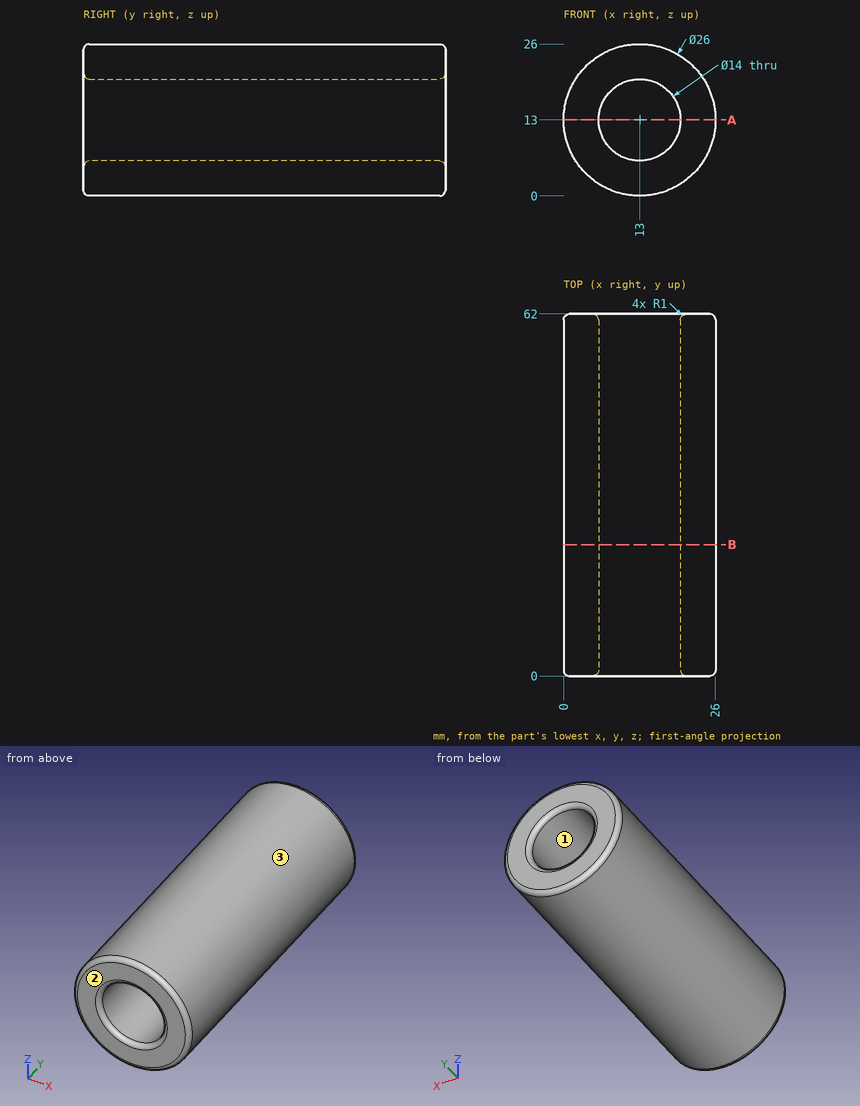
The figure shows three views and two pictorial views of one solid part (mm, origin at its lowest corner). Answer the questions. Coordinates: 2 decimals unless noted, no trailing zeros. Order: outer loops, then holes, each group sorted by start corner. A loop starts at its lowest first (then second) coordinate and runs counter-clockwise, first axis right, second up. Notation, with made-up numbers: M 89.25,-36 L 109.25,-36 A29 cw 109.25,-9 Z; hole C 58,39.5 d8. An arc over 180 degrees is marked long. Use CSV: the item, a comma, the result in double quotes.
1) Section B-B on y = 22.5 is taken. Write down the section's boundary in (x, z).
Worked out:
outline,"C 13,13 d26; hole C 13,13 d14"
2) Flat-ended cylindrical pins translate along their axes: pin 1 Ø10 at (y, z) = (38.5, 22.5) entering from -X; pin 2 Ø8 at (x, y) = (23.5, 45.5) entering from -Z; pin 3 Ø8 at (x, y) = (18.5, 21.5) entering from -Z; pin 4 Ø10 at (y, z) = (22, 16.5) entering from -X. Find the tip coordinate at first contact, or state that the pin passes through.
Worked out:
pin 1,"stops at x = 0.8"
pin 2,"stops at z = 1.74"
pin 3,"stops at z = 0.09"
pin 4,"stops at x = 0"
3) Determine the mould class of the marked faces 1, 2 and 3 for opening direction X: released by +X, released by -X, zero draft, split by the parting line, or undercut.
Worked out:
face 1,"undercut"
face 2,"zero draft"
face 3,"split by the parting line"
4) Section A-A on z = 13 is taken. Write down the section's boundary in (x, y).
Worked out:
outline,"M 0,1 A1 ccw 1,0 L 5,0 A1 ccw 6,1 L 6,61 A1 ccw 5,62 L 1,62 A1 ccw 0,61 Z; M 20,1 A1 ccw 21,0 L 25,0 A1 ccw 26,1 L 26,61 A1 ccw 25,62 L 21,62 A1 ccw 20,61 Z"
5) Consider line 1 (X direction, y = 48.5, z = 13); line 2 (X direction, y = 23, z = 8.25); line 3 (Z direction, x = 9.75, y = 34). Determine where each line is inside the solid, lowest interval first. Write a range as [from, to].
Worked out:
line 1,"x = [0, 6], [20, 26]"
line 2,"x = [0.9, 7.86], [18.14, 25.1]"
line 3,"z = [0.41, 6.8], [19.2, 25.59]"
